For this review, take the finished solid that the model builds, in its own axes (mm). Face numbers are marked on the shaded views. A direction names the side the tool comes from. Coordinates: 2 decimals unless noted, no trailing zeros. Loops run counter-clockwise (first coordinate to the right, second up) from the corner with the lowest first, then second, coordinate; pieces in that order, holes last.
1. Mouldability with a two-part tool opening along X and no side actions: class the marked faces 1, 2 and 3 as pulls with the +X half, pulls with the -X half, needs draft (parallel to the pull), parting line crosses it, or undercut.
2. To check wall thickness, follow probe 1 along X at (y, z) = (0.5, 2); probe 2 along Y at (x, z) = (-5.5, -2.25); probe 3 along X at (y, z) = (-4, -2.5). State the ranges of each line that lie inside material, in increasing order.
3. Take a section at C-C, the plane x = -7. State the section outline as (y, z) points (3 decimals).
4. Take a section at B-B, the plane z = -2.5. State the section outline as (x, y) points.
5. Machinability: for the marked faces 4 and 5, which of the approach directions +Z, -Z, +X, -X, +Y, -Y give a long, thin tool a straight path to every point of the face, cutting with its end or side? Answer none if there is none.
6. Clearance check with flat-ended pins moving along their axes: P1, Ø2, axis at x = -10, y = 7, coming from the +Z side; P2, Ø1, axis at y = 8, z = 1.5, coming from the +X side. State where each tip first meets the part, or that it passes through.
7. Take a section at D-D, the plane x = 14. State the section outline as (y, z) points (3 decimals), then the cut area to 3 significant figures.
8. Take a section at A-A, the plane y = 0. State the section outline as (x, z) points (3 decimals).
```python
from build123d import *

# Parameters (mm, degrees)
SKETCH1_R           = 19.05
BOSS_EXTRUDE1_DEPTH = 3.175


with BuildPart() as part:
    # Sketch1 → Boss-Extrude1 (new body, symmetric)
    with BuildSketch(Plane.XY):
        Circle(SKETCH1_R)
        Polygon((0, 14.664696837), (-12.7, 7.332348419), (-12.7, -7.332348419), (0, -14.664696837), (12.7, -7.332348419), (12.7, 7.332348419), align=None, mode=Mode.SUBTRACT)
    extrude(amount=BOSS_EXTRUDE1_DEPTH, both=True)


solid = part.part
```
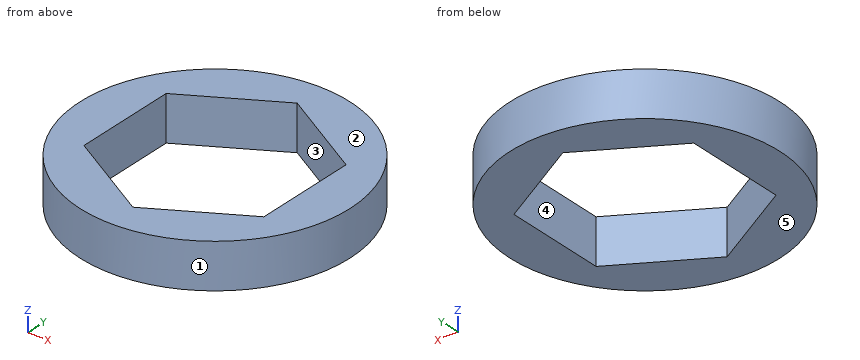
Results list:
1. face 1: parting line crosses it
1. face 2: needs draft
1. face 3: undercut
2. probe 1: x = -19.04 to -12.7, 12.7 to 19.04
2. probe 2: y = -18.24 to -11.49, 11.49 to 18.24
2. probe 3: x = -18.63 to -12.7, 12.7 to 18.63
3. outline: (-17.717, -3.175) - (-10.623, -3.175) - (-10.623, 3.175) - (-17.717, 3.175) - close; (10.623, -3.175) - (17.717, -3.175) - (17.717, 3.175) - (10.623, 3.175) - close
4. outline: circle Ø38.1 at (0, 0); hole (-12.7, -7.33) - (0, -14.66) - (12.7, -7.33) - (12.7, 7.33) - (0, 14.66) - (-12.7, 7.33) - close
5. face 4: +Z, -Z
5. face 5: -Z, +X, -X, +Y, -Y
6. P1: passes through
6. P2: stops at x = 17.51
7. outline: (-12.919, -3.175) - (12.919, -3.175) - (12.919, 3.175) - (-12.919, 3.175) - close
7. area: 164 mm2
8. outline: (-19.05, -3.175) - (-12.7, -3.175) - (-12.7, 3.175) - (-19.05, 3.175) - close; (12.7, -3.175) - (19.05, -3.175) - (19.05, 3.175) - (12.7, 3.175) - close
